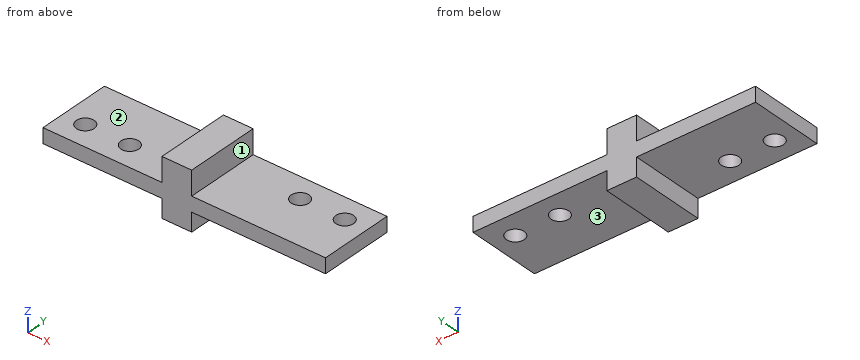
from build123d import *

# Parameters (mm, degrees)
F1_DEPTH = 31.75
F3_D     = 7.62


with BuildPart() as f1:
    # F0 (on Front) → F1 (new body)
    with BuildSketch(Plane.XZ):
        Polygon((0, 6.35), (0, 0), (50.8, 0), (50.8, -7.9248), (63.5, -7.9248), (63.5, 0), (120.65, 0), (120.65, 6.35), (63.5, 6.35), (63.5, 16.6624), (50.8, 16.6624), (50.8, 6.35), align=None)
    extrude(amount=F1_DEPTH)

    # F3 (through all)
    with Locations(Plane(origin=(0, 0, 0), x_dir=(1, 0, 0), z_dir=(0, 0, -1))):
        with Locations((9.525, 21.4376), (28.575, 21.4376), (92.075, 10.3124), (111.125, 10.3124)):
            Hole(F3_D / 2)


solid = f1.part
Work out the finished part from the listing and answer in its coordinate system (mm). Face numbers are marked on the shaded views. A direction names the side the tool comes from. Coordinates: 2 decimals unless noted, no trailing zeros. Write each loop counter-clockwise with the first axis right and the second up, starting at its lowest first coordinate (ties: lowest second). Pieces come first, ordered by that corner, then holes.
1. For the marked faces 1, 2 and 3, determine the directions among +Z, -Z, +X, -X, +Y, -Y from which every point of the face is accessible in a straight line to the end or side of a thin tool.
Results list:
face 1: +Z, +X, +Y, -Y
face 2: +Z, -X, +Y, -Y
face 3: -Z, +X, +Y, -Y
2. Flat-ended cylindrical pins translate along their axes: pin 1 (16 mm diameter, centred on x = 92, y = -23, fed in from -Z); pin 2 (4 mm diameter, centred on y = -22, z = -5, fed in from +X); pin 3 (12 mm diameter, centred on x = 28.58, y = -21.44, fed in from +Z). Find the tip coordinate at first contact, or state that the pin passes through.
Results list:
pin 1: stops at z = 0
pin 2: stops at x = 63.5
pin 3: stops at z = 6.35
3. The part is cut by section A-A, the plane x = 27. Write down the section's boundary in (y, z), and give its area (3 significant figures).
Results list:
outline: (-31.75, 0) - (-24.91, 0) - (-24.91, 6.35) - (-31.75, 6.35) - close; (-17.97, 0) - (0, 0) - (0, 6.35) - (-17.97, 6.35) - close
area: 158 mm2
4. The part is cut by section C-C, the plane z = 2.25. Write down the section's boundary in (x, y) (3 decimals).
Results list:
outline: (0, -31.75) - (120.65, -31.75) - (120.65, 0) - (0, 0) - close; hole circle Ø7.62 at (9.525, -21.438); hole circle Ø7.62 at (28.575, -21.438); hole circle Ø7.62 at (92.075, -10.312); hole circle Ø7.62 at (111.125, -10.312)
5. The part is cut by section D-D, the plane y = -16.5. Write down the section's boundary in (x, z).
Results list:
outline: (0, 0) - (50.8, 0) - (50.8, -7.92) - (63.5, -7.92) - (63.5, 0) - (120.65, 0) - (120.65, 6.35) - (63.5, 6.35) - (63.5, 16.66) - (50.8, 16.66) - (50.8, 6.35) - (0, 6.35) - close
6. Consider line 1 along Y through (x, z) = (111, 5); line 2 along X through (y, z) = (-7, 2); line 3 along Z through (x, y) = (92, -16.5). Determine where each line is inside the solid, lowest interval first.
Results list:
line 1: y = -31.75 to -14.12, -6.5 to 0
line 2: x = 0 to 90.19, 93.96 to 109.24, 113.01 to 120.65
line 3: z = 0 to 6.35
7. The part is cut by section B-B, the plane y = -9. Write down the section's boundary in (x, z), and give its area (3 significant figures).
Results list:
outline: (0, 0) - (50.8, 0) - (50.8, -7.92) - (63.5, -7.92) - (63.5, 0) - (88.5, 0) - (88.5, 6.35) - (63.5, 6.35) - (63.5, 16.66) - (50.8, 16.66) - (50.8, 6.35) - (0, 6.35) - close; (95.65, 0) - (107.55, 0) - (107.55, 6.35) - (95.65, 6.35) - close; (114.7, 0) - (120.65, 0) - (120.65, 6.35) - (114.7, 6.35) - close
area: 907 mm2
